Check sheet for the modelled part. Datum: model origin and axes. Units: mm. Face numbers are marked on the shaded views. Give positions to 0.01 mm unless a question says otherwise; leave off trailing zeros. Order: outer loops, then holes, each group sorted by start corner. A loop starts at its lowest first (then second) coordinate and runs counter-clockwise, first axis right, second up. Notation, with made-up numbers: M -13,-22.5 L 11,-22.5 A18 ccw 11,12.5 Z; hole C 58.25,-32.5 d1. An arc over 180 degrees is marked long. Return JSON: item names as keys, results as strings. Group by question number.
from build123d import *

# Parameters (mm, degrees)
BOSS_EXTRU_1_DEPTH = 25
BOSS_EXTRU_2_DEPTH = 1
BOSS_EXTRU_3_START = -1
BOSS_EXTRU_3_DEPTH = 1
ESQUISSE6_R        = 5
BOSS_EXTRU_4_DEPTH = 2
ESQUISSE7_R        = 2.5
BOSS_EXTRU_5_DEPTH = 2


with BuildPart() as part:
    # Esquisse1 → Boss.-Extru.1 (new body)
    with BuildSketch(Plane(origin=(0, 0, 0), x_dir=(1, 0, 0), z_dir=(0, 1, 0))):
        Polygon((-3.234042553, -21.946808511), (-2.234042553, -21.946808511), (-2.234042553, 7.275558935), (47.765957447, 7.275558935), (47.765957447, -21.946808511), (48.765957447, -21.946808511), (48.765957447, 8.053191489), (-3.234042553, 8.053191489), align=None)
    extrude(amount=BOSS_EXTRU_1_DEPTH)

    # Esquisse3 → Boss.-Extru.2 (add)
    with BuildSketch(Plane.ZY.offset(3.234042553)):
        with BuildLine():
            Line((21.946808511, 25), (21.946808511, 0))
            ThreePointArc((21.946808511, 0), (34.446808511, 12.5), (21.946808511, 25))
        make_face()
    extrude(amount=-BOSS_EXTRU_2_DEPTH)

    # Esquisse4 → Boss.-Extru.3 (add)
    with BuildSketch(Plane(origin=(48.765957447, 0, 0), x_dir=(0, 0, -1), z_dir=(1, 0, 0)).offset(BOSS_EXTRU_3_START)):
        with BuildLine():
            Line((-21.946808511, 25), (-21.946808511, 0))
            ThreePointArc((-21.946808511, 0), (-34.446808511, 12.5), (-21.946808511, 25))
        make_face()
    extrude(amount=BOSS_EXTRU_3_DEPTH)

    # Esquisse6 → Boss.-Extru.4 (add)
    with BuildSketch(Plane(origin=(-2.234042553, 0, 0), x_dir=(0, 0, -1), z_dir=(1, 0, 0))):
        with Locations(Location((-21.946808511, 12.22196254, 0), (0, 0, 180))):
            Circle(ESQUISSE6_R)
    extrude(amount=BOSS_EXTRU_4_DEPTH)

    # Esquisse7 → Boss.-Extru.5 (add)
    with BuildSketch(Plane(origin=(-0.234042553, 0, 0), x_dir=(0, 0, -1), z_dir=(1, 0, 0))):
        with Locations((-21.946808511, 12.22196254)):
            Circle(ESQUISSE7_R)
    extrude(amount=BOSS_EXTRU_5_DEPTH)


solid = part.part
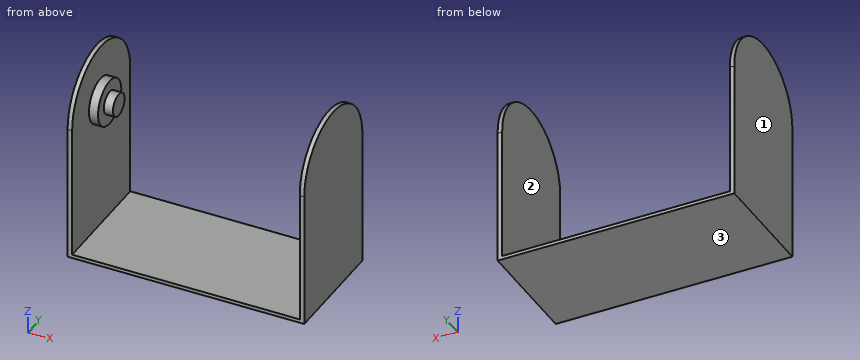
1) Sectioned sample at C-C on z = 25.5. Record the boundary of the cut face in (x, y), then the cut area to 3 significant figures.
2) Depth check by flat-ended pin: P1, Ø1, axis at x = 10, y = 12, coming from the +Z side. Enter the tip coordinate at first touch or a pass-through.
3) Sectioned sample at D-D on x = 25. Record the boundary of the cut face in (y, z), then the cut area to 3 significant figures.
4) Sectioned sample at B-B on y = 23. Record the boundary of the cut face in (x, z), then the cut area to 3 significant figures.
5) Material ranges on line 1 along X through (y, z) = (14.75, 26.5); line 2 along Z through (x, y) = (6, 4); line 3 along Y through (x, z) = (-1, 24), recorded low to high.
6) Sectioned sample at A-A on z = 7. Record the boundary of the cut face in (x, y).
7) Release check for a two-part mould opening along X. For the marked faces 1, 2 and 3 record: released by +X, released by -X, zero draft, split by the parting line, or undercut.
Reply:
{
 "1": {"outline": "M -3.23,0.52 L -2.23,0.52 L -2.23,8.7 L -0.23,8.7 L -0.23,15.74 L -2.23,15.74 L -2.23,24.48 L -3.23,24.48 Z; M 47.77,0.52 L 48.77,0.52 L 48.77,24.48 L 47.77,24.48 Z", "area": "62.0 mm^2"},
 "2": {"P1": "z = -7.28"},
 "3": {"outline": "M 0,-8.05 L 25,-8.05 L 25,-7.28 L 0,-7.28 Z", "area": "19.4 mm^2"},
 "4": {"outline": "M -3.23,-8.05 L 48.77,-8.05 L 48.77,28.73 L 47.77,28.73 L 47.77,-7.28 L -2.23,-7.28 L -2.23,28.73 L -3.23,28.73 Z", "area": "112 mm^2"},
 "5": {"line 1": "-3.23 to -2.23, 47.77 to 48.77", "line 2": "-8.05 to -7.28", "line 3": "7.66 to 16.78"},
 "6": {"outline": "M -3.23,0 L -2.23,0 L -2.23,25 L -3.23,25 Z; M 47.77,0 L 48.77,0 L 48.77,25 L 47.77,25 Z"},
 "7": {"face 1": "released by -X", "face 2": "undercut", "face 3": "zero draft"}
}
